Could you check a few things on this model? Use its own coordinates, in mm. Face numbers are marked on the shaded views. Give positions to 0.01 mm unless a question says otherwise; leave off trailing zeros. Loops run counter-clockwise (first coordinate to the right, second up) from the corner with the lowest first, then second, coordinate; pieces in that order, holes last. Notation, with made-up numbers: M 12.5,6.5 L 45.5,6.5 A23 cw 45.5,18.5 Z; hole C 66.25,65 d3. An arc over 180 degrees is marked long. Use CSV: the item, a comma, the result in double quotes.
```python
from build123d import *

# Parameters (mm, degrees)
SKETCH1_W           = 38
SKETCH1_H           = 12
BOSS_EXTRUDE1_DEPTH = 1.2
SKETCH2_W           = 26.6
SKETCH2_H           = 7.62
BOSS_EXTRUDE2_DEPTH = 1.2
SKETCH3_W           = 22.38
SKETCH3_H           = 5.58
CUT_EXTRUDE1_DEPTH  = 0.1
SKETCH4_R           = 0.5
CUT_EXTRUDE2_DEPTH  = 20.960961901


with BuildPart() as part:
    # Sketch1 → Boss-Extrude1 (new body)
    with BuildSketch(Plane(origin=(0, 0, 0), x_dir=(1, 0, 0), z_dir=(0, 1, 0))):
        Rectangle(SKETCH1_W, SKETCH1_H)
    extrude(amount=BOSS_EXTRUDE1_DEPTH)

    # Sketch2 → Boss-Extrude2 (add)
    with BuildSketch(Plane(origin=(0, 1.2, 0), x_dir=(1, 0, 0), z_dir=(0, 1, 0))):
        with Locations((-1.81, 0.41)):
            Rectangle(SKETCH2_W, SKETCH2_H)
    extrude(amount=BOSS_EXTRUDE2_DEPTH)

    # Sketch3 → Cut-Extrude1 (cut)
    with BuildSketch(Plane(origin=(0, 2.4, 0), x_dir=(1, 0, 0), z_dir=(0, 1, 0))):
        with Locations((-1.81, 0)):
            Rectangle(SKETCH3_W, SKETCH3_H)
    extrude(amount=-CUT_EXTRUDE1_DEPTH, mode=Mode.SUBTRACT)

    # Sketch4 → Cut-Extrude2 (cut, through all)
    with BuildSketch(Plane(origin=(0, 1.2, 0), x_dir=(1, 0, 0), z_dir=(0, 1, 0))):
        with Locations(Location((-16.948688295, 3.981018796, 0), (0, 0, 270))):
            Circle(SKETCH4_R)
        with Locations(Location((-16.948688295, 1.441018796, 0), (0, 0, 270))):
            Circle(SKETCH4_R)
        with Locations(Location((-16.948688295, -1.098981204, 0), (0, 0, 270))):
            Circle(SKETCH4_R)
        with Locations(Location((-16.948688295, -3.638981204, 0), (0, 0, 270))):
            Circle(SKETCH4_R)
    extrude(amount=-CUT_EXTRUDE2_DEPTH, mode=Mode.SUBTRACT)


solid = part.part
```
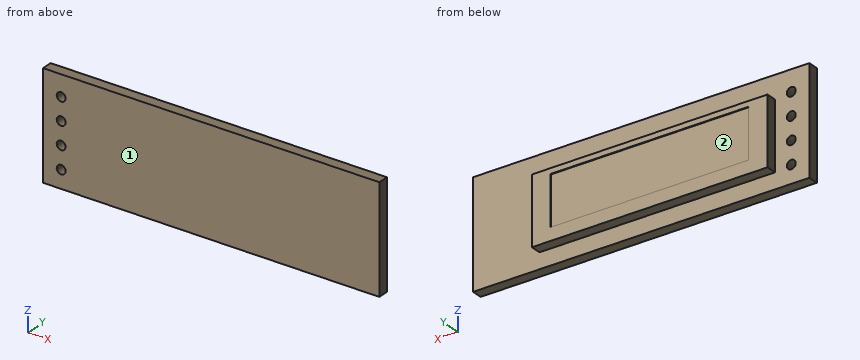
1. I'm going to push flat-ended pins straight in: pin 1 Ø0.6 at (x, y) = (-1, 2) entering from -Z; pin 2 Ø0.6 at (y, z) = (2, 1) entering from +X; pin 3 Ø0.6 at (x, y) = (4, 2) entering from +Z. Where does each tip first touch, or does it pass through?
Outcome:
pin 1,"z = -4.22"
pin 2,"x = 11.49"
pin 3,"z = 3.4"
2. I want a section at B-B, the plane y = 1.6. List the corners of the cut face in (x, z) for me, then the cut area to 3 significant figures.
Outcome:
outline,"M -15.11,-4.22 L 11.49,-4.22 L 11.49,3.4 L -15.11,3.4 Z"
area,"203 mm2"
3. I want a section at C-C, the plane x = 14. List the corners of the cut face in (y, z) for me.
Outcome:
outline,"M 0,-6 L 1.2,-6 L 1.2,6 L 0,6 Z"
4. I want a section at A-A, the plane x = -10.5. List the corners of the cut face in (y, z) for me.
Outcome:
outline,"M 0,-6 L 1.2,-6 L 1.2,-4.22 L 2.4,-4.22 L 2.4,-2.79 L 2.3,-2.79 L 2.3,2.79 L 2.4,2.79 L 2.4,3.4 L 1.2,3.4 L 1.2,6 L 0,6 Z"
5. Please list where these lines run through material, in increasing order: line 1 (Z direction, x = -17, y = 1.15); line 2 (X direction, y = 0.6, z = -1.5); line 3 (Y direction, x = 17, z = -1.5).
Outcome:
line 1,"-6 to -4.48, -3.48 to -1.94, -0.94 to 0.6, 1.6 to 3.14, 4.14 to 6"
line 2,"-19 to -17.45, -16.45 to 19"
line 3,"0 to 1.2"
6. If we mould it in two halves opening along X, with no side actions, what happens to the marked faces 1 and 2? For each: +X half, -X half, draft (parallel to the pull), parting line (faces both ways), or undercut.
Outcome:
face 1,"draft"
face 2,"undercut"
